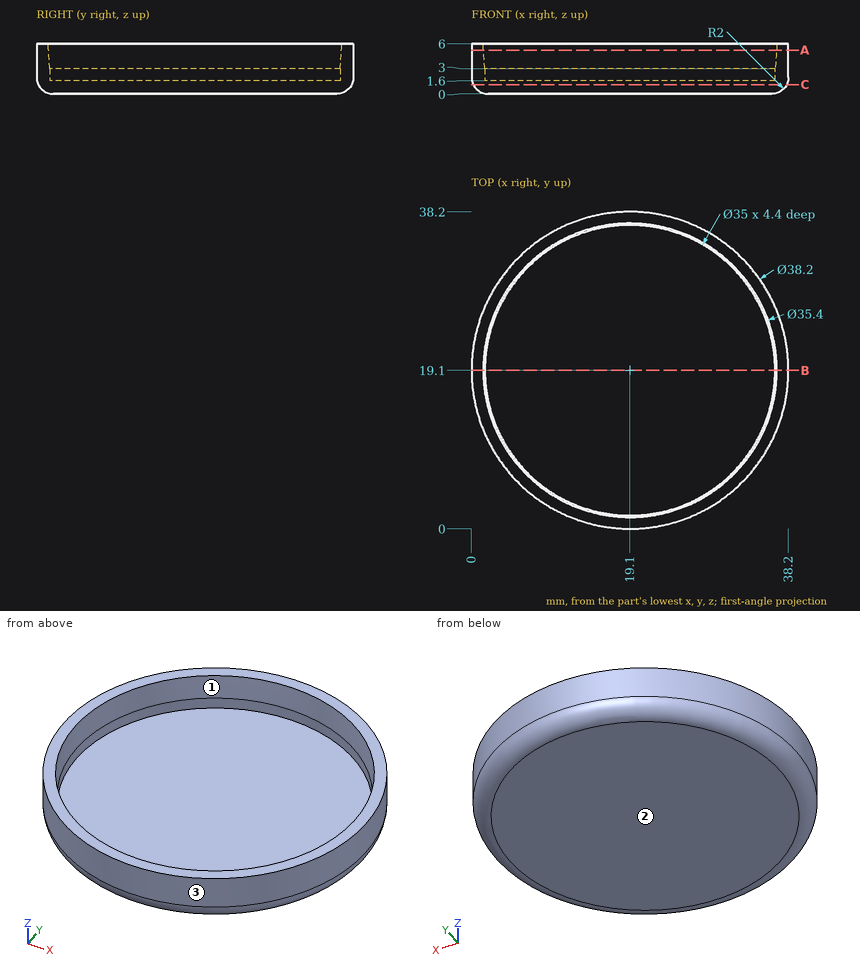
Job drawing, mm, ordinate dimensions from the low corner. One solid piece. Round coordinates to 2 decimals unless told otherwise and drop trailing zeros. Loops run counter-clockwise (first coordinate to the right, second up) from the corner with the lowest first, then second, coordinate; pieces in that order, holes last. Notation, with made-up numbers: (-5.75, 46) -> (7.25, 46) arc R14 ccw to (7.25, 64) -> close; hole circle Ø8 at (9.5, 5). An arc over 180 degrees is marked (long way). Use CSV: the item, a comma, the result in double quotes. Start each with the question number.
Q1. Saw through at C-C on z = 1.1. Give the cut face in (x, y).
Q2. Flat gauge pins, fed straight in: pin 1 Ø1 at (x, z) = (11, 1.5) entering from +Y; pin 2 Ø8 at (x, y) = (7.5, 30.5) entering from -Z; pin 3 Ø3 at (x, z) = (34, 1.5) entering from +Y; pin 4 Ø1 at (x, y) = (25, 7) entering from +Z. Where does each tip first touch, or does it go through?
Q3. Mould opens along X. For the marked faces 1, 2 and 3 say: +X half, -X half, draft (parallel to the pull), parting line (faces both ways), or undercut.
Q4. Saw through at B-B on y = 19.1. Give the cut face in (x, z).
Q5. Drill centre lines: L1, parallel to Y at x = 19.1, z = 2.6; L2, parallel to Z at x = 7.5, y = 13; L3, parallel to Y at x = 6, z = 4. Where is each one in solid material? Low to high.
Q6. Saw through at A-A on z = 5.25. Give the cut face in (x, y), and give its area (3 significant figures).
Solutions:
1,outline,"circle Ø37.77 at (19.1, 19.1)"
2,pin 1,"stops at y = 36.58"
2,pin 2,"stops at z = 0"
2,pin 3,"stops at y = 32.67"
2,pin 4,"stops at z = 1.6"
3,face 1,"undercut"
3,face 2,"draft"
3,face 3,"parting line"
4,outline,"(0, 2) arc R2 ccw to (2, 0) -> (36.2, 0) arc R2 ccw to (38.2, 2) -> (38.2, 6) -> (36.8, 6) -> (36.6, 3) -> (36.6, 1.6) -> (1.6, 1.6) -> (1.6, 3) -> (1.4, 6) -> (0, 6) -> close"
5,L1,"y = 0 to 1.6, 36.6 to 38.2"
5,L2,"z = 0 to 1.6"
5,L3,"y = 5.2 to 7.4, 30.8 to 33"
6,outline,"circle Ø38.2 at (19.1, 19.1); hole circle Ø35.3 at (19.1, 19.1)"
6,area,"167 mm^2"
